Verification items for the finished model (mm, model axes). Face numbers are marked on the shaded views. A direction names the side the tool comes from. Coordinates: 2 decimals unless noted, no trailing zeros. Order: outer loops, then holes, each group sorted by start corner. A loop starts at its lowest first (then second) coordinate and runs counter-clockwise, first axis right, second up. Notation, with made-up numbers: (27, -7) -> (45, -7) arc R20 ccw to (45, 31) -> close; hole circle Ø11 at (-9, -7). An arc over 180 degrees is marked (long way). Answer as CSV lines item,"result".
```python
from build123d import *

# Parameters (mm, degrees)
SKETCH1_R                 = 37
BOSS_EXTRUDE1_DEPTH       = 5
SKETCH2_R                 = 9.25
SKETCH2_R_2               = 2.25
BOSS_EXTRUDE2_DEPTH       = 7
F_1_0MM_DOWEL_HOLE1_D     = 3
F_1_0MM_DOWEL_HOLE1_DEPTH = 8
CUT_EXTRUDE1_START        = -2
SKETCH5_R                 = 2.25
CUT_EXTRUDE1_DEPTH        = 2
CUT_EXTRUDE2_DEPTH        = 2.5


with BuildPart() as part:
    # Sketch1 → Boss-Extrude1 (new body)
    with BuildSketch(Plane(origin=(0, 0, 0), x_dir=(1, 0, 0), z_dir=(0, 1, 0))):
        with Locations(Location((0, 0, 0), (0, 0, 270))):
            Circle(SKETCH1_R)
    extrude(amount=BOSS_EXTRUDE1_DEPTH)

    # Sketch2 → Boss-Extrude2 (add)
    with BuildSketch(Plane(origin=(0, 5, 0), x_dir=(1, 0, 0), z_dir=(0, 1, 0))):
        with Locations(Location((0, 0, 0), (0, 0, 270))):
            Circle(SKETCH2_R)
        with Locations(Location((0, 0, 0), (0, 0, 270))):
            Circle(SKETCH2_R_2, mode=Mode.SUBTRACT)
    extrude(amount=BOSS_EXTRUDE2_DEPTH)

    # Ø1.0mm Dowel Hole1
    with Locations(Plane.ZY.offset(9.25)):
        with Locations((0, 8)):
            Hole(F_1_0MM_DOWEL_HOLE1_D / 2, depth=F_1_0MM_DOWEL_HOLE1_DEPTH)

    # Sketch5 → Cut-Extrude1 (cut)
    with BuildSketch(Plane(origin=(0, 5, 0), x_dir=(1, 0, 0), z_dir=(0, 1, 0)).offset(CUT_EXTRUDE1_START)):
        with Locations(Location((0, 0, 0), (0, 0, 270))):
            Circle(SKETCH5_R)
    extrude(amount=CUT_EXTRUDE1_DEPTH, mode=Mode.SUBTRACT)

    # Sketch6 → Cut-Extrude2 (cut)
    with BuildSketch(Plane(origin=(-6.5, 0, 0), x_dir=(0, 0, -1), z_dir=(1, 0, 0))):
        Polygon((-2.75, 12), (-2.75, 6.41228676), (0, 4.824573519), (2.75, 6.41228676), (2.75, 12), align=None)
    extrude(amount=CUT_EXTRUDE2_DEPTH, mode=Mode.SUBTRACT)


solid = part.part
```
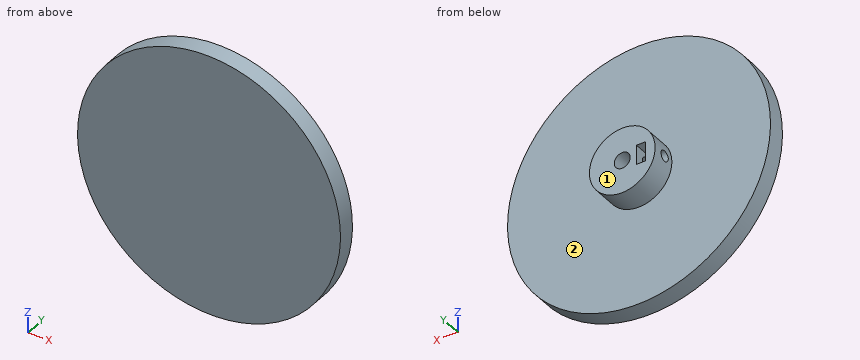
Item 1: Thickness scan on line 1 (Y direction, x = -7.1, z = 0); line 2 (Y direction, x = -18.5, z = -12); line 3 (Z direction, x = -8.35, y = 8). Record the ranges inside material, lowest first.
Answer list:
line 1,"0 to 6.5, 9.5 to 12"
line 2,"0 to 5"
line 3,"-3.98 to -1.5, 1.5 to 3.98"
Item 2: Section check A-A, the plane x = 0. Record the boundary of the cut face in (y, z), plus the area to 3 significant figures.
Answer list:
outline,"(0, -37) -> (5, -37) -> (5, -9.25) -> (12, -9.25) -> (12, -2.25) -> (3, -2.25) -> (3, 2.25) -> (12, 2.25) -> (12, 9.25) -> (5, 9.25) -> (5, 37) -> (0, 37) -> close"
area,"459 mm2"
Item 3: Section check C-C, the plane z = 7.5. Record the boundary of the cut face in (x, y), plus the area to 3 significant figures.
Answer list:
outline,"(-36.23, 0) -> (36.23, 0) -> (36.23, 5) -> (5.41, 5) -> (5.41, 12) -> (-5.41, 12) -> (-5.41, 5) -> (-36.23, 5) -> close"
area,"438 mm2"
Item 4: Section check D-D, the plane z = -7. Record the boundary of the cut face in (x, y), plus the area to 3 significant figures.
Answer list:
outline,"(-36.33, 0) -> (36.33, 0) -> (36.33, 5) -> (6.05, 5) -> (6.05, 12) -> (-6.05, 12) -> (-6.05, 5) -> (-36.33, 5) -> close"
area,"448 mm2"
Item 5: Section check B-B, the plane y = 10.5. Record the boundary of the cut face in (x, z).
Answer list:
outline,"circle Ø18.5 at (0, 0); hole (-6.5, -2.75) -> (-4, -2.75) -> (-4, 2.75) -> (-6.5, 2.75) -> close; hole circle Ø4.5 at (0, 0)"
Item 6: Tool access check on the marked faces 1 and 2. Record the directions out of +Z, -Z, +X, -X, +Y, -Y that give a thin tool (end or side, any length) a straight path to the whole face; none if there is none.
Answer list:
face 1,"+Z, -Z, +X, -X, +Y"
face 2,"+Y"
Item 7: Depth check by flat-ended pin: pin 1 Ø1.5 at (y, z) = (9, 9) entering from +X; pin 2 Ø8 at (x, z) = (-9.5, 14.5) entering from +Y; pin 3 Ø1 at (y, z) = (10, -5.5) entering from +X. Enter the tip coordinate at first touch or a pass-through.
Answer list:
pin 1,"x = 4.18"
pin 2,"y = 5"
pin 3,"x = 7.78"
